```python
from build123d import *

# Parameters (mm, degrees)
F2_R     = 15.5
F3_DEPTH = 2150.001


with BuildPart() as f1:
    # F0 (on Front) → F1 (revolve)
    with BuildSketch(Plane.XZ):
        Polygon((940, 100), (-940, 100), (-940, 275), (-950, 275), (-950, 200), (-1150, 200), (-1200, 160), (-1200, 0), (1200, 0), (1200, 160), (1150, 200), (950, 200), (950, 275), (940, 275), align=None)
    revolve(axis=Axis((0, 0, 0), (1, 0, 0)))

    # F2 (on face) → F3 (cut, through all)
    with BuildSketch(Plane.YZ.offset(950)):
        with Locations((0, 240)):
            Circle(F2_R)
        with Locations((-169.705627, 169.705627)):
            Circle(F2_R)
        with Locations((-240, 0)):
            Circle(F2_R)
        with Locations((-169.705627, -169.705627)):
            Circle(F2_R)
        with Locations((0, -240)):
            Circle(F2_R)
        with Locations((169.705627, -169.705627)):
            Circle(F2_R)
        with Locations((240, 0)):
            Circle(F2_R)
        with Locations((169.705627, 169.705627)):
            Circle(F2_R)
    extrude(amount=-F3_DEPTH, mode=Mode.SUBTRACT)


solid = f1.part
```
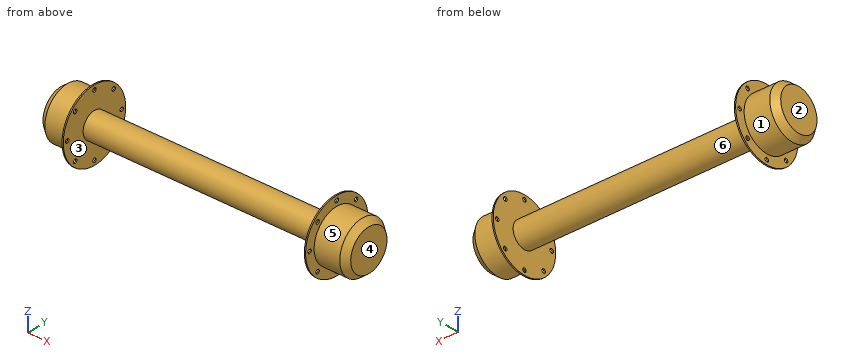
Check sheet for the modelled part. Datum: model origin and axes. Units: mm. Face numbers are marked on the shaded views. A direction names the side the tool comes from. Give positions to 0.01 mm unless a question says otherwise; leave off trailing zeros. Loops run counter-clockwise (first coordinate to the right, second up) from the corner with the lowest first, then second, coordinate; pieces in that order, holes last. Notation, with made-up numbers: (64, 54.5) - (84, 54.5) arc R25 cw to (84, 69.5) - close; hole circle Ø1 at (47.5, 35). An arc over 180 degrees is marked (long way). One line per question, with ' | ' between items. Start each with the question number.
1. Gauge pin test, flat ends, axial feed: pin 1 Ø6 at (x, z) = (-257, -84.5) entering from -Y; pin 2 Ø4 at (x, y) = (-928, -4.5) entering from -Z; pin 3 Ø2 at (x, y) = (-508.5, 67.5) entering from -Z. Record the tip position at first contact, or that the pin passes through.
2. Draft check along X on the marked faces 1, 2, 3 and 4. Enter one of: released by +X, released by -X, zero draft, split by the parting line, or undercut.
3. Cross-section at A-A, the plane x = 1007. Enter the section's corners in (y, z), plus the area to 3 significant figures.
4. Set-up check for the marked faces 5 and 6: record each of +Z, -Z, +X, -X, +Y, -Y from which the full face is reachable in a straight line by a thin tool's end or side.
5. Cross-section at B-B, the plane x = 484.5. Enter the section's corners in (y, z).
6. Material ranges on line 1 along X through (y, z) = (203.5, 6.5); line 2 along X through (y, z) = (-12, -153); line 3 along Z through (x, y) = (943.75, 0), recorded low to high. Write a range as [from, to].
Check result:
1) pin 1: stops at y = -57.95 | pin 2: stops at z = -99.97 | pin 3: stops at z = -74.68
2) face 1: zero draft | face 2: released by -X | face 3: undercut | face 4: released by +X
3) outline: circle Ø400 at (0, 0) | area: 126,000 mm2
4) face 5: +X | face 6: none
5) outline: circle Ø200 at (0, 0)
6) line 1: x = [-950, -940], [940, 950] | line 2: x = [-1200, -940], [940, 1200] | line 3: z = [-275, -255.5], [-224.5, 224.5], [255.5, 275]
